Input: part model. Units: mm. Frame: model coordinates. A direction names the side the tool comes from. Coordinates: 2 decimals unless noted, no trailing zeros. Write each loop counter-clockwise with the first axis right and the second up, starting at its lowest first coordinate (ties: lowest second). Pieces come first, ordered by that corner, then holes. Notation, with made-up numbers: M 0,38.5 L 10,38.5 A30 cw 10,71.5 Z; hole C 43,33 d1. An arc over 180 degrees is marked long. Use CSV: the item, a comma, the result in double quotes.
```python
from build123d import *

# Parameters (mm, degrees)
SKETCH2_W                                      = 50.8
SKETCH2_H                                      = 25.4
BOSS_EXTRUDE1_DEPTH                            = 1.5875
SKETCH3_W                                      = 1.5875
SKETCH3_H                                      = 25.4
BOSS_EXTRUDE2_DEPTH                            = 6.35
FILLET1_R                                      = 0.508
LPATTERN1_COUNT                                = 14
LPATTERN1_PITCH                                = 3.7846
FILLET1_OF_LPATTERN1_R                         = 0.508
CBORE_FOR_4_SOCKET_HEAD_CAP_SCREW1_D           = 3.2639
CBORE_FOR_4_SOCKET_HEAD_CAP_SCREW1_CBORE_D     = 5.55752
CBORE_FOR_4_SOCKET_HEAD_CAP_SCREW1_CBORE_DEPTH = 6.35


with BuildPart() as part:
    # Sketch2 → Boss-Extrude1 (new body)
    with BuildSketch(Plane(origin=(0, 0, 0), x_dir=(1, 0, 0), z_dir=(0, 1, 0))):
        with Locations((4.112380952, -1.952517007)):
            Rectangle(SKETCH2_W, SKETCH2_H)
    extrude(amount=BOSS_EXTRUDE1_DEPTH)

    # Sketch3 → Boss-Extrude2 (add)
    with BuildSketch(Plane(origin=(0, 1.5875, 0), x_dir=(1, 0, 0), z_dir=(0, 1, 0))):
        with Locations((-20.493869048, -1.952517007)):
            Rectangle(SKETCH3_W, SKETCH3_H)
    boss_extrude2 = extrude(amount=BOSS_EXTRUDE2_DEPTH)

    # Fillet1
    fillet1_edges = [part.edges().sort_by_distance(p)[0] for p in [
        (-20.493869048, 7.9375, -10.747482993),
        (-21.287619048, 7.9375, 1.952517007),
        (-20.493869048, 7.9375, 14.652517007),
        (-19.700119048, 7.9375, 1.952517007),
    ]]
    fillet(fillet1_edges, radius=FILLET1_R)

    # LPattern1: Boss-Extrude2 ×14
    with Locations(*[(i * LPATTERN1_PITCH, 0, 0) for i in range(1, LPATTERN1_COUNT)]):
        add(boss_extrude2)

    # Fillet1 of LPattern1
    fillet1_of_lpattern1_edges = [part.edges().sort_by_distance(p)[0] for p in [
        (-16.709269048, 7.9375, -10.747482993),
        (-17.503019048, 7.9375, 1.952517007),
        (-16.709269048, 7.9375, 14.652517007),
        (-15.915519048, 7.9375, 1.952517007),
        (-12.924669048, 7.9375, -10.747482993),
        (-13.718419048, 7.9375, 1.952517007),
        (-12.924669048, 7.9375, 14.652517007),
        (-12.130919048, 7.9375, 1.952517007),
        (-9.140069048, 7.9375, -10.747482993),
        (-9.933819048, 7.9375, 1.952517007),
        (-9.140069048, 7.9375, 14.652517007),
        (-8.346319048, 7.9375, 1.952517007),
        (-5.355469048, 7.9375, -10.747482993),
        (-6.149219048, 7.9375, 1.952517007),
        (-5.355469048, 7.9375, 14.652517007),
        (-4.561719048, 7.9375, 1.952517007),
        (-1.570869048, 7.9375, -10.747482993),
        (-2.364619048, 7.9375, 1.952517007),
        (-1.570869048, 7.9375, 14.652517007),
        (-0.777119048, 7.9375, 1.952517007),
        (2.213730952, 7.9375, -10.747482993),
        (1.419980952, 7.9375, 1.952517007),
        (2.213730952, 7.9375, 14.652517007),
        (3.007480952, 7.9375, 1.952517007),
        (5.998330952, 7.9375, -10.747482993),
        (5.204580952, 7.9375, 1.952517007),
        (5.998330952, 7.9375, 14.652517007),
        (6.792080952, 7.9375, 1.952517007),
        (9.782930952, 7.9375, -10.747482993),
        (8.989180952, 7.9375, 1.952517007),
        (9.782930952, 7.9375, 14.652517007),
        (10.576680952, 7.9375, 1.952517007),
        (13.567530952, 7.9375, -10.747482993),
        (12.773780952, 7.9375, 1.952517007),
        (13.567530952, 7.9375, 14.652517007),
        (14.361280952, 7.9375, 1.952517007),
        (17.352130952, 7.9375, -10.747482993),
        (16.558380952, 7.9375, 1.952517007),
        (17.352130952, 7.9375, 14.652517007),
        (18.145880952, 7.9375, 1.952517007),
        (21.136730952, 7.9375, -10.747482993),
        (20.342980952, 7.9375, 1.952517007),
        (21.136730952, 7.9375, 14.652517007),
        (21.930480952, 7.9375, 1.952517007),
        (24.921330952, 7.9375, -10.747482993),
        (24.127580952, 7.9375, 1.952517007),
        (24.921330952, 7.9375, 14.652517007),
        (25.715080952, 7.9375, 1.952517007),
        (28.705930952, 7.9375, -10.747482993),
        (27.912180952, 7.9375, 1.952517007),
        (28.705930952, 7.9375, 14.652517007),
        (29.499680952, 7.9375, 1.952517007),
    ]]
    fillet(fillet1_of_lpattern1_edges, radius=FILLET1_OF_LPATTERN1_R)

    # CBORE for #4 Socket Head Cap Screw1 (through all)
    with Locations(Plane(origin=(-8.597783115, 7.9375, 1.952517007), x_dir=(0, 0, 1), z_dir=(0, 1, 0))):
        with Locations((0, 0), (0, 25.407628135)):
            CounterBoreHole(CBORE_FOR_4_SOCKET_HEAD_CAP_SCREW1_D / 2, CBORE_FOR_4_SOCKET_HEAD_CAP_SCREW1_CBORE_D / 2, CBORE_FOR_4_SOCKET_HEAD_CAP_SCREW1_CBORE_DEPTH)


solid = part.part
```
1. Section A-A (y = 2.5). State how many separate pieces and enclosed holes the cut face has, then the cut area to 3 significant figures.
Resolved:
separate pieces,"16"
enclosed holes,"0"
area,"546 mm^2"
2. Access query for faces 4 (the flat face through (4, 0, 2)), 5 (the flat face through (3.007, 4, 2)). Directions: +Z, -Z, +X, -X, +Y, -Y. A direction counts if a zero-diameter tool reaches every point of the face in a straight line with its end or side. Return the directions, or none.
Resolved:
face 4,"+Z, -Z, +X, -X, -Y"
face 5,"+Z, -Z, +Y"
3. Material intervals for line 1 (Y direction, x = 23.5, z = -4.25); line 2 (Y direction, x = 14, z = -0.25), sorted ascending. Write a range as [from, to].
Resolved:
line 1,"y = [0, 1.59]"
line 2,"y = [0, 7.92]"
4. Mould query, pull axis Z, two halves, no side actions, for faces 1 (the cylindrical face through (17.366, 4.807, 4.675)), 2 (the cylindrical face through (15.217, 0.783, 2.306)), 3 (the flat face through (-3, 1.588, 2)). Classes: pulls with the +Z half, pulls with the -Z half, needs draft (parallel to the pull), parting line crosses it, or undercut.
Resolved:
face 1,"undercut"
face 2,"undercut"
face 3,"needs draft"
5. Contact query for flat-ended pins moving along their axis: pin 1 Ø2.5 at (x, z) = (11.5, 7.5) entering from +Y; pin 2 Ø4.5 at (y, z) = (4.5, -2.5) entering from +X; pin 3 Ø12 at (x, z) = (-16, -8) entering from -Y. Output: stop coordinate, or through.
Resolved:
pin 1,"stops at y = 7.9"
pin 2,"stops at x = 29.5"
pin 3,"stops at y = 0"
6. Section C-C (x = 23). Return loops of the section in (y, z).
Resolved:
outline,"M 0,-10.75 L 1.59,-10.75 L 1.59,14.65 L 0,14.65 Z"
